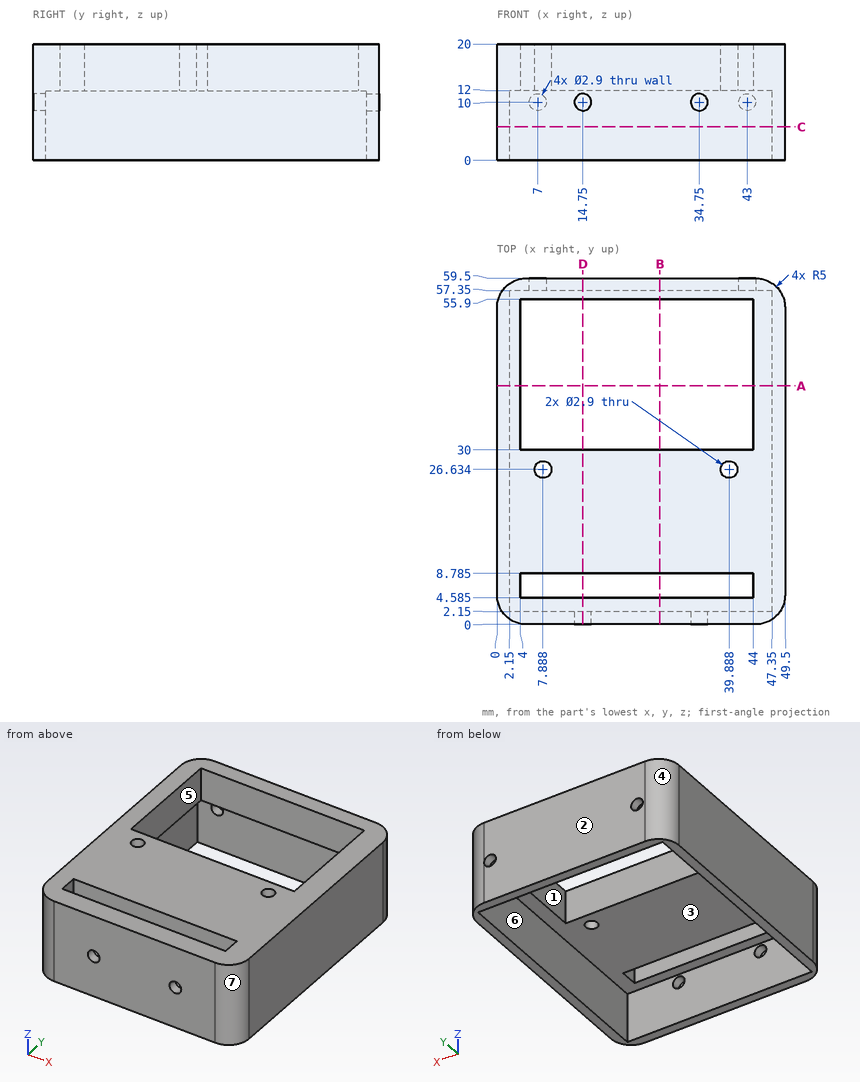
Verification items for this drawing (mm, ordinates from the low corner). A direction names the side the tool comes from. Give positions to 0.01 mm unless a question says otherwise; leave off trailing zeros. Loops run counter-clockwise (first coordinate to the right, second up) from the corner with the lowest first, then second, coordinate; pieces in that order, holes last.
1. Go/stop test with flat-tipped pins: P1, Ø1, axis at x = 15, z = 10.5, coming from the -Y side; P2, Ø3.5, axis at x = 7.888, y = 26.634, coming from the -Z side; P3, Ø6, axis at x = 40, y = 52, coming from the -Z side. Record where each tip stops, or that it passes through.
Derived:
P1: stops at y = 57.35
P2: stops at z = 12
P3: passes through
2. Material ranges on probe 1 along Y at (x, z) = (14, 18.5) (3 decimals); probe 2 along Z at (x, y) = (7, 58); probe 3 along Y at (x, z) = (26, 8), recorded low to high.
Derived:
probe 1: y = 0 to 4.585, 8.785 to 30, 55.9 to 59.5
probe 2: z = 0 to 8.55, 11.45 to 20
probe 3: y = 0 to 2.15, 57.35 to 59.5
3. Release check for a two-part mould opening along X. For the marked faces 4, 5, 6 and 7 record: +X half, -X half, draft (parallel to the pull), parting line (faces both ways), or undercut.
Derived:
face 4: -X half
face 5: undercut
face 6: undercut
face 7: +X half
4. Cross-section at C-C on z = 5.75. Record the cut outline in (x, y).
Derived:
outline: (0, 5) arc R5 ccw to (5, 0) - (44.5, 0) arc R5 ccw to (49.5, 5) - (49.5, 54.5) arc R5 ccw to (44.5, 59.5) - (5, 59.5) arc R5 ccw to (0, 54.5) - close; hole (2.15, 2.15) - (47.35, 2.15) - (47.35, 57.35) - (2.15, 57.35) - close
5. Tool access check on the marked faces 1, 2 and 3. Record the directions out of +Z, -Z, +X, -X, +Y, -Y that give a thin tool (end or side, any length) a straight path to the whole face; none if there is none.
Derived:
face 1: +Z, -Z
face 2: +Z, -Z, +X, -X, +Y
face 3: -Z
6. Cross-section at B-B on x = 28. Record the cut outline in (y, z) (3 decimals), and give its area (3 significant figures).
Derived:
outline: (0, 0) - (2.15, 0) - (2.15, 12) - (4.585, 12) - (4.585, 20) - (0, 20) - close; (8.785, 12) - (30, 12) - (30, 20) - (8.785, 20) - close; (55.9, 12) - (57.35, 12) - (57.35, 0) - (59.5, 0) - (59.5, 20) - (55.9, 20) - close
area: 287 mm2
7. Cross-section at D-D on x = 14.75. Record the cut outline in (y, z) (3 decimals).
Derived:
outline: (0, 0) - (2.15, 0) - (2.15, 8.55) - (0, 8.55) - close; (0, 11.45) - (2.15, 11.45) - (2.15, 12) - (4.585, 12) - (4.585, 20) - (0, 20) - close; (8.785, 12) - (30, 12) - (30, 20) - (8.785, 20) - close; (55.9, 12) - (57.35, 12) - (57.35, 0) - (59.5, 0) - (59.5, 20) - (55.9, 20) - close
8. Cross-section at A-A on y = 41. Record the cut outline in (x, z).
Derived:
outline: (0, 0) - (2.15, 0) - (2.15, 12) - (4, 12) - (4, 20) - (0, 20) - close; (44, 12) - (47.35, 12) - (47.35, 0) - (49.5, 0) - (49.5, 20) - (44, 20) - close
